Autodesk Inventor part; units mm, degrees
ref_plane "YZ Plane" through (0, 0, 0) normal (1, 0, 0) x (0, 1, 0)
ref_plane "XZ Plane" through (0, 0, 0) normal (0, 1, 0) x (-1, 0, 0)
ref_plane "XY Plane" through (0, 0, 0) normal (0, 0, 1) x (1, 0, 0)
sketch "スケッチ1" plane through (0, 0, 0) normal (0, 1, 0) x (-1, 0, 0)
  line L0 (0, 0) -> (106, 0)
  line L1 (106, 0) -> (106, -120)
  line L2 (106, -120) -> (0, -120)
  line L3 (0, -120) -> (0, 0)
  dimension "d0" = 106
  dimension "d1" = 120
extrude "押し出し1" add sketch "スケッチ1" along normal blind 3
sketch "スケッチ4" plane through (0, 3, 0) normal (0, 1, 0) x (1, 0, 0)
  line L0 (-106, 120) -> (-106, 0)
  line L1 (-106, 5) -> (0, 5)
  line L2 (0, 0) -> (0, 120)
  line L3 (-120, 115) -> (0, 115)
  line L4 (-106, 0) -> (0, 0)
  line L5 (0, 120) -> (-106, 120)
  line L6 (-106, 0) -> (0, 0)
  line L7 (-101, 0) -> (-101, 120)
  line L8 (-5, 120) -> (-5, 0)
  point P0 (-101, 5)
  point P1 (-5, 5)
  point P2 (-5, 115)
  point P3 (-101, 115)
  dimension "d22" = 5
  dimension "d23" = 5
  dimension "d24" = 5
  dimension "d25" = 5
hole "穴2" at (-101, 3, -5) at (-5, 3, -5) at (-5, 3, -115) at (-101, 3, -115) direction (0, -1, 0) diameter 3.2 end through all
sketch "スケッチ5" plane through (0, 3, 0) normal (0, 1, 0) x (1, 0, 0)
  line L0 (-106, 120) -> (-106, 0)
  line L1 (-106, 60) -> (0, 60)
  line L2 (0, 0) -> (0, 120)
  point P0 (-53, 60)
hole "穴3" at (-53, 3, -60) direction (0, -1, 0) diameter 10 end through all
equation "\"d38\" = Thickness"
equation "\"BendRadius\" = Thickness"
equation "\"BendReliefWidth\" = Thickness"
equation "\"BendReliefDepth\" = 0.5 * Thickness"
equation "\"CornerReliefSize\" = 4 * Thickness"
equation "\"MinimumRemnant\" = 2 * Thickness"
equation "\"TransitionRadius\" = BendRadius"
equation "\"JacobiRadiusSize\" = BendRadius"
equation "\"GapSize\" = Thickness"
properties part number "link2_plate3" material "アルミニウム 6061"
For this review, take the finished solid that the model builds, in its own axes (mm). Round coordinates to 2 decimals unless told otherwise and drop trailing zeros. Write each loop counter-clockwise with the first axis right and the second up, starting at its lowest first coordinate (ties: lowest second). Pieces come first, ordered by that corner, then holes. Notation, with made-up numbers: (42, 30.5) - (91, 30.5) arc R24 ccw to (91, 61.5) - close; hole circle Ø4 at (9.5, -13.75). An arc over 180 degrees is marked (long way). Answer as a JSON object with one key per item and string values.
1. For pin 1 Ø6 at (x, z) = (-53, -60) entering from -Y, flat-tipped, find the tip position at first contact; note if it passes through.
Response values:
{"pin 1": "passes through"}
2. We need section B-B on z = -115. Give the boundary of the cut face in (x, y).
Response values:
{"outline": "(-106, 0) - (-102.6, 0) - (-102.6, 3) - (-106, 3) - close; (-99.4, 0) - (-6.6, 0) - (-6.6, 3) - (-99.4, 3) - close; (-3.4, 0) - (0, 0) - (0, 3) - (-3.4, 3) - close"}
3. We need section D-D on x = -53. Give the boundary of the cut face in (y, z), then the cut area to 3 significant figures.
Response values:
{"outline": "(0, -120) - (3, -120) - (3, -65) - (0, -65) - close; (0, -55) - (3, -55) - (3, 0) - (0, 0) - close", "area": "330 mm2"}
4. Draft analysis for pull direction Z (two halves, no side actions). For faces 1 (the face through (-64, 0, -59)), 2 (the face through (-57.957, 1.479, -60.651)), 3 (the face through (-5.481, 1.479, -113.474)), 4 (the face through (-52, 1, 0)), state which applies: +Z half, -Z half, draft (parallel to the pull), parting line (faces both ways), or undercut.
Response values:
{"face 1": "draft", "face 2": "undercut", "face 3": "undercut", "face 4": "+Z half"}
5. We need section A-A on x = -101. Give the boundary of the cut face in (y, z), then the cut area to 3 significant figures.
Response values:
{"outline": "(0, -120) - (3, -120) - (3, -116.6) - (0, -116.6) - close; (0, -113.4) - (3, -113.4) - (3, -6.6) - (0, -6.6) - close; (0, -3.4) - (3, -3.4) - (3, 0) - (0, 0) - close", "area": "341 mm2"}
6. We need section C-C on z = -60. Give the boundary of the cut face in (x, y), then the cut area to 3 significant figures.
Response values:
{"outline": "(-106, 0) - (-58, 0) - (-58, 3) - (-106, 3) - close; (-48, 0) - (0, 0) - (0, 3) - (-48, 3) - close", "area": "288 mm2"}
7. To check wall thickness, follow line 1 along X through (y, z) = (1.05, -5); line 2 along Z through (x, y) = (-5, 2.15); line 3 along Z through (x, y) = (-6, 2.4). State the ranges of each line that lie inside material, in increasing order.
Response values:
{"line 1": "x = -106 to -102.6, -99.4 to -6.6, -3.4 to 0", "line 2": "z = -120 to -116.6, -113.4 to -6.6, -3.4 to 0", "line 3": "z = -120 to -116.25, -113.75 to -6.25, -3.75 to 0"}
